Model file for the job. Use its own axes, mm. Coordinates: 2 decimals unless noted, no trailing zeros. Write each loop counter-clockwise with the first axis right and the second up, starting at its lowest first coordinate (ties: lowest second). Pieces come first, ordered by that corner, then holes. Notation, with made-up numbers: (0.5, 13.5) - (58.5, 13.5) arc R33 cw to (58.5, 45.5) - close; hole circle Ø2 at (73, 72.25). An arc over 180 degrees is marked (long way). Put each result on its own line as item: value. Start each with the question number.
1. Drill centre lines: L1, parallel to X at y = 0, z = -4.15; L2, parallel to Z at x = -27, y = 0. Where is each one in solid material? Low to high. Write a range as from..to.
2. Saw through at A-A, the plane y = 0. Write the cut outline in (x, z), plus the area to 3 significant figures.
3. Saw through at D-D, the plane x = 17. Write the cut outline in (y, z), plus the area to 3 significant figures.
4. Drop flat-ended pins along their axis: P1, Ø5, axis at y = -3.5, z = -0.5, coming from the +X side; P2, Ø2.5, axis at x = -40.5, y = 0, coming from the -Z side; P3, Ø2, axis at x = -26.5, y = -3.5, coming from the +Z side. Give the stop position or say it passes through.
5. Saw through at C-C, the plane x = -40.5. Write the cut outline in (y, z), plus the area to 3 significant figures.
6. Saw through at B-B, the plane z = 0. Write the cut outline in (x, y).
```python
from build123d import *

# Parameters (mm, degrees)
SKETCH_1_R               = 5
SKETCH_1_R_2             = 4
EXTRUDE_1_DEPTH          = 46.5
SKETCH_2_R               = 1.5
CUT_EXTRUDE_1_DEPTH      = 6
CUT_EXTRUDE_1_DEPTH_BACK = 6


with BuildPart() as part:
    # 草图1 → 凸台-拉伸1 (new body, symmetric)
    with BuildSketch(Plane(origin=(0, 0, 0), x_dir=(0, 0, -1), z_dir=(1, 0, 0))):
        Circle(SKETCH_1_R)
        Circle(SKETCH_1_R_2, mode=Mode.SUBTRACT)
    extrude(amount=EXTRUDE_1_DEPTH, both=True)

    # 草图2 → 切除-拉伸1 (cut, two sides)
    with BuildSketch(Plane.XY) as cut_extrude_1_sk:
        with Locations((40.5, 0)):
            Circle(SKETCH_2_R)
        with Locations((-40.5, 0)):
            Circle(SKETCH_2_R)
    extrude(amount=CUT_EXTRUDE_1_DEPTH, mode=Mode.SUBTRACT)
    extrude(cut_extrude_1_sk.sketch, amount=-CUT_EXTRUDE_1_DEPTH_BACK, mode=Mode.SUBTRACT)


solid = part.part
```
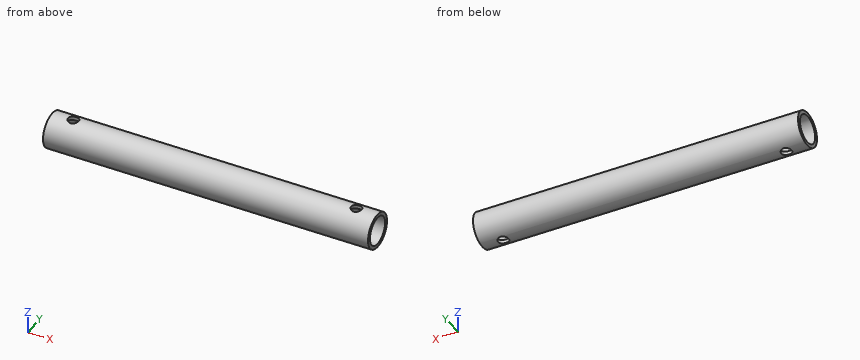
Final values:
1. L1: x = -46.5..-42, -39..39, 42..46.5
1. L2: z = -5..-4, 4..5
2. outline: (-46.5, -5) - (-42, -5) - (-42, -4) - (-46.5, -4) - close; (-46.5, 4) - (-42, 4) - (-42, 5) - (-46.5, 5) - close; (-39, -5) - (39, -5) - (39, -4) - (-39, -4) - close; (-39, 4) - (39, 4) - (39, 5) - (-39, 5) - close; (42, -5) - (46.5, -5) - (46.5, -4) - (42, -4) - close; (42, 4) - (46.5, 4) - (46.5, 5) - (42, 5) - close
2. area: 174 mm²
3. outline: circle Ø10 at (0, 0); hole circle Ø8 at (0, 0)
3. area: 28.3 mm²
4. P1: stops at x = 46.5
4. P2: passes through
4. P3: stops at z = 4.33
5. outline: (-1.5, -4.77) - (-1.5, -3.71) arc R4 cw to (-1.5, 3.71) - (-1.5, 4.77) arc R5 ccw to start; (1.5, -4.77) arc R5 ccw to (1.5, 4.77) - (1.5, 3.71) arc R4 cw to (1.5, -3.71) - close
5. area: 22.2 mm²
6. outline: (-46.5, -5) - (46.5, -5) - (46.5, -4) - (-46.5, -4) - close; (-46.5, 4) - (46.5, 4) - (46.5, 5) - (-46.5, 5) - close
